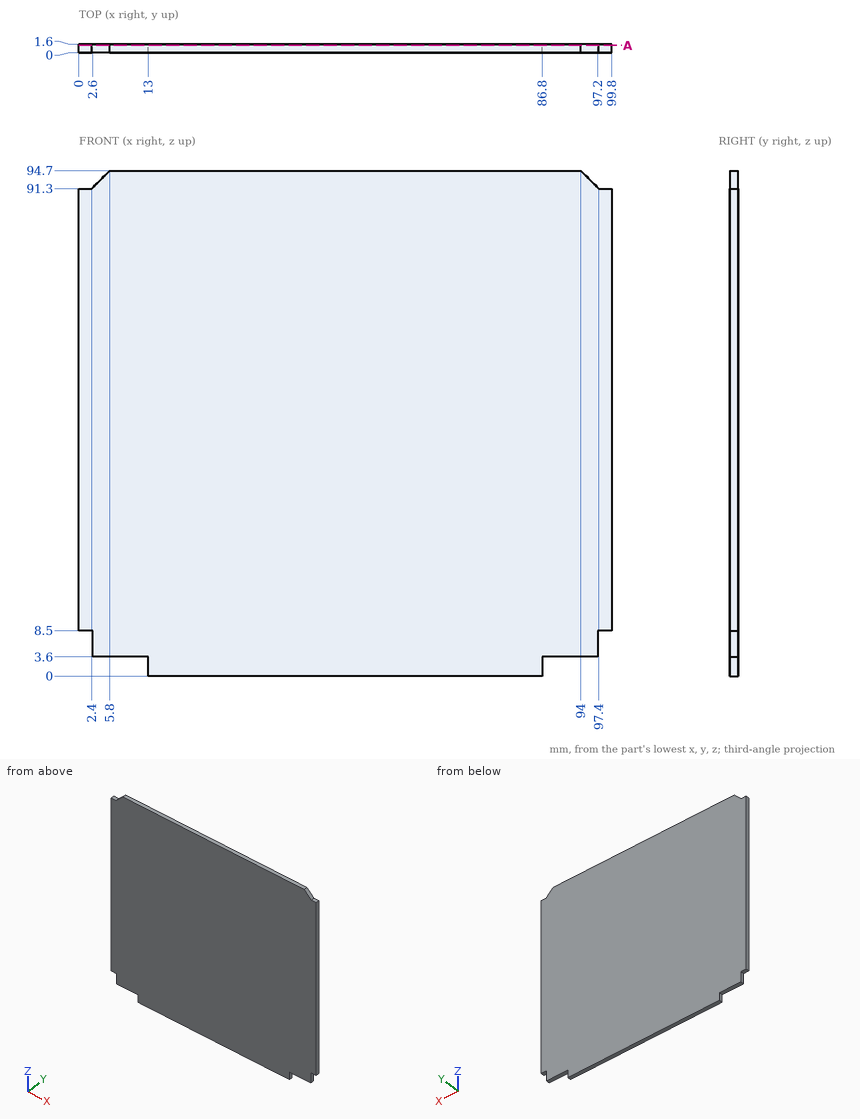
Study the drawing (mm; zero at the part's minimum x, y, z) and answer. Round coordinates to 2 decimals unless told otherwise and drop trailing zeros. Write each loop counter-clockwise with the first axis right and the second up, starting at its lowest first coordinate (ties: lowest second). Pieces come first, ordered by that corner, then holes. Notation, with made-up numbers: (-8.5, 55.25) - (22.5, 55.25) arc R16 cw to (22.5, 84.25) - close; hole circle Ø4 at (-35, 58). An arc over 180 degrees is marked (long way). Use a Markdown table: item, result. Add a question column.
1. Flat-ended cylindrical pins translate along their axes: P1, Ø0.8, axis at x = 8, y = 1, coming from the -Z side; P2, Ø0.5, axis at x = 1, y = 1, coming from the -Z side; P3, Ø0.8, axis at y = 1, z = 1.5, coming from the +X side. Find the tip coordinate at first contact, or state that the pin passes through.
2. Consider line 1 (Z direction, x = 88.5, y = 0.3); line 2 (X direction, y = 1.5, z = 7.5); line 3 (Z direction, x = 5.5, y = 0.2). Determine where each line is inside the solid, lowest interval first.
3. The part is cut by section A-A (y = 1.35). Write down the section's boundary in (x, z).
Reported:
| question | item | result |
|---|---|---|
| 1 | P1 | z = 3.6 |
| 1 | P2 | z = 8.5 |
| 1 | P3 | x = 86.8 |
| 2 | line 1 | 3.6 to 94.7 |
| 2 | line 2 | 2.6 to 97.2 |
| 2 | line 3 | 3.6 to 94.4 |
| 3 | outline | (0, 8.5) - (2.6, 8.5) - (2.6, 3.6) - (13, 3.6) - (13, 0) - (86.8, 0) - (86.8, 3.6) - (97.2, 3.6) - (97.2, 8.5) - (99.8, 8.5) - (99.8, 91.3) - (97.4, 91.3) - (94, 94.7) - (5.8, 94.7) - (2.4, 91.3) - (0, 91.3) - close |
